Check sheet for the modelled part. Datum: model origin and axes. Units: mm. A direction names the side the tool comes from. Round coordinates to 2 decimals unless told otherwise and drop trailing zeros. Order: outer loops, then holes, each group sorted by start corner. A loop starts at its lowest first (then second) coordinate and runs counter-clockwise, first axis right, second up.
Autodesk Inventor part; units mm, degrees
ref_plane "Work Plane1" through (0, -2.4764, 0) normal (-1, 0, 0) x (0, 0, 1)
ref_plane "YZ Plane" through (0, 0, 0) normal (1, 0, 0) x (0, 1, 0)
ref_plane "XZ Plane" through (0, 0, 0) normal (0, 1, 0) x (-1, 0, 0)
sketch "Sketch1" plane through (0, 0, 0) normal (0, 0, 1) x (1, 0, 0)
  circle A0 centre (0, -2.4764) radius 2.5 construction
  line L0 (-0.39, 0.0236) -> (0, 0.0236) construction
  line L1 (-3.206, 0) -> (3.4858, 0)
  line L2 (-1.7872, -3.2564) -> (1.7872, -3.2564) construction
  arc A1 (-1.847, -1.8509) -> (-1.7872, -3.2564) centre (0, -2.4764) ccw
  line L3 (0, 1.949) -> (0, -3.4788)
  arc A2 (-0.39, -0.1364) -> (0.39, -0.1364) centre (0, -0.1364) ccw
  arc A3 (3.3844, -5.047) -> (-3.3844, -5.047) centre (0, -2.4764) ccw
  line L4 (-2.34, -1.6964) -> (-1.9578, -1.6964)
  line L5 (-0.39, -0.1364) -> (-0.39, 0.2425)
  arc A4 (-0.78, 0.5446) -> (-2.7529, -1.0081) centre (0, -2.4764) ccw
  arc A5 (-0.39, 0.2425) -> (-0.78, 0.5446) centre (-0.702, 0.2425) ccw
  arc A6 (-2.7529, -1.0081) -> (-2.34, -1.6964) centre (-2.34, -1.2284) ccw
  arc A7 (-1.847, -1.8509) -> (-1.9578, -1.6964) centre (-1.9578, -1.8134) ccw
  line L6 (0, 1.7736) -> (2.5298, 1.7736) construction
  line L7 (-1.7872, -3.2564) -> (-2.3673, -4.889)
  arc A8 (-3.3844, -5.047) -> (-2.3673, -4.889) centre (-2.9185, -4.6932) ccw
  line L8 (0, -0.5264) -> (-1.2778, -0.5264) construction
  line L9 (1.7872, -3.2564) -> (2.3673, -4.889)
  arc A9 (2.3673, -4.889) -> (3.3844, -5.047) centre (2.9185, -4.6932) ccw
  arc A10 (1.7872, -3.2564) -> (1.847, -1.8509) centre (0, -2.4764) ccw
  line L10 (2.34, -1.6964) -> (1.9578, -1.6964)
  line L11 (0.39, -0.1364) -> (0.39, 0.2425)
  arc A11 (2.7529, -1.0081) -> (0.78, 0.5446) centre (0, -2.4764) ccw
  arc A12 (0.78, 0.5446) -> (0.39, 0.2425) centre (0.702, 0.2425) ccw
  arc A13 (2.34, -1.6964) -> (2.7529, -1.0081) centre (2.34, -1.2284) ccw
  arc A14 (1.9578, -1.6964) -> (1.847, -1.8509) centre (1.9578, -1.8134) ccw
  point P0 (0.39, 0.0236)
  dimension "d0" = 5
  dimension "d3" = 0.78
  dimension "d4" = 0.39
  dimension "d5" = 8.5
  dimension "d8" = 3.12
  dimension "d9" = 0.78
  dimension "d10" = 0.312
  dimension "d11" = 0.468
  dimension "d12" = 0.117
  dimension "d13" = 0.585
  dimension "d14" = 1.95
  dimension "d15" = 1.95
extrude "Body" add sketch "Sketch1" along normal blind 0.6 contours A4 A6 L4 A7 A1 L7 A8 A3 L3 L1 L5 A5 | L1 L3 A2 L5 | L3 A3 L1 A11 A12 L11 | L1 L11 A2 L3 | L1 A3 A9 L9 A10 A14 L10 A13 A11
ref_plane "Work Plane1" through (0, -2.4764, 0) normal (-1, 0, 0) x (0, 0, 1)
equation "\"d0\" = WD"
equation "\"d3\" = 0.2 * ND"
equation "\"d4\" = 0.1 * ND"
equation "\"d5\" = SD2"
equation "\"d8\" = 0.8 * ND"
equation "\"d9\" = 0.2 * ND"
equation "\"d10\" = 0.08 * ND"
equation "\"d11\" = 0.12 * ND"
equation "\"d12\" = 0.03 * ND"
equation "\"d13\" = 0.15 * ND"
equation "\"d14\" = 0.5 * ND"
equation "\"d15\" = 0.5 * ND"
equation "\"d16\" = SD"
equation "\"ND\" = 3.9"
equation "\"SD\" = 0.6"
equation "\"WD\" = WDMIN"
equation "\"d1\" = 1.6 * ND"
equation "\"d2\" = ND"
equation "\"SD2\" = 8.5"
equation "\"d6\" = ND"
equation "\"d7\" = 0.15 * ND"
equation "\"WDMIN\" = 5"
equation "\"SNB\" = 0.7"
equation "\"WDMAX\" = 6"
equation "\"BUBRMI\" = 1.1"
properties part number "ANSI B27.7 - 5, E" material "Steel, Mild"
Item 1: Sectioned sample at C-C (x = 0). Record the cut outline in (y, z), and give its area (3 significant figures).
Answer:
outline: (-0.53, 0) - (1.77, 0) - (1.77, 0.6) - (-0.53, 0.6) - close
area: 1.38 mm2
Item 2: Access from +Z, -Z, +X, -X, +Y, -Y to the whole of each face (thin tool, end or side, straight path). Record for faces 4 (the cylindrical face through (-1.9, 0, 0.3)), 5 (the flat face through (0, 0, 0.6)).
Answer:
face 4: +Z, -Z
face 5: +Z, +X, -X, +Y, -Y
Item 3: Scan lines: line 1 along X through (y, z) = (-2.5, 0.4); line 2 along X through (y, z) = (-1, 0.4); line 3 along Y through (x, z) = (1.5, 0.2). Record each from-to range of solid material in increasing order.
Answer:
line 1: x = -4.25 to -1.95, 1.95 to 4.25
line 2: x = -3.99 to -2.75, 2.75 to 3.99
line 3: y = 0.26 to 1.5
Item 4: Sectioned sample at A-A (y = -1.5). Record the cut outline in (x, z).
Answer:
outline: (-4.14, 0) - (-2.72, 0) - (-2.72, 0.6) - (-4.14, 0.6) - close; (2.72, 0) - (4.14, 0) - (4.14, 0.6) - (2.72, 0.6) - close
Item 5: Sectioned sample at D-D (x = 1). Record the cut outline in (y, z), and give its area (3 significant figures).
Answer:
outline: (0.48, 0) - (1.65, 0) - (1.65, 0.6) - (0.48, 0.6) - close
area: 0.705 mm2
Item 6: Release check for a two-part mould opening along X. For faces 1 (the cylindrical face through (-0.13, 1.77, 0.3)), 2 (the cylindrical face through (1.9, 0, 0.3)), 3 (the flat face through (0, 0, 0)) record: released by +X, released by -X, zero draft, split by the parting line, or undercut.
Answer:
face 1: split by the parting line
face 2: undercut
face 3: zero draft
